Work out the finished part from the listing and answer in its coordinate system (mm). Face numbers are marked on the shaded views. A direction names the side the tool comes from. Give positions to 0.01 mm unless a question says otherwise; leave off trailing zeros. Write item = value, one per line. Start each with the question number.
1. Flat-ended cylindrical pins translate along their axes: pin 1 Ø4 at (x, z) = (34.5, -5) entering from +Y; pin 2 Ø8 at (x, y) = (35.5, -1.5) entering from +Z; pin 3 Ø4 at (x, y) = (33.5, 3) entering from +Z; pin 4 Ø8 at (y, z) = (-5.5, 0.5) entering from +X. Find the tip coordinate at first contact, or state that the pin passes through.
2. For the marked faces 1 and 2, determine the directions among +Z, -Z, +X, -X, +Y, -Y from which every point of the face is accessible in a straight line to the end or side of a thin tool.
3. Consider L1, parallel to X at y = 4, z = -2; L2, parallel to Z at x = 51, y = -3; L3, parallel to Y at x = 27, z = -5.25. Determine where each line is inside the solid, lowest interval first. Write a range as [from, to].
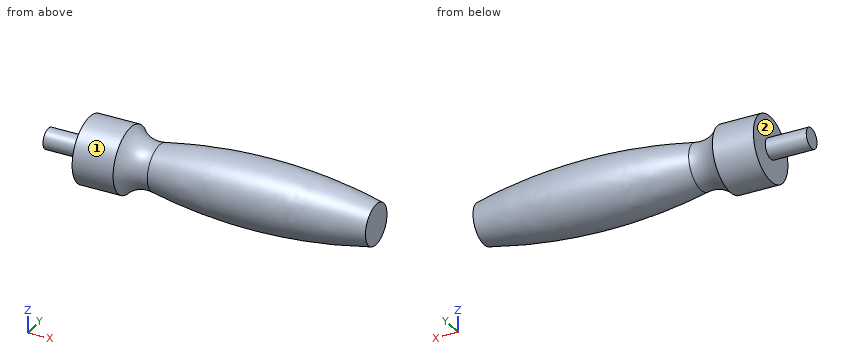
```python
from build123d import *

# Parameters (mm, degrees)
F0_W = 10
F0_H = 2.5


# Not quite as in the source:
# - a fillet or chamfer that OpenCascade refuses, or shapes differently, is made with other operations: its cross-section is extruded or revolved along the edge and cut away or added


with BuildPart() as f1:
    # F0 (on Front) → F1 (revolve)
    with BuildSketch(Plane.XZ):
        with Locations((-5, 1.25)):
            Rectangle(F0_W, F0_H)
        Polygon((0, 8), (0, 2.5), (0, 0), (10, 0), (10, 4), (10, 8), align=None)
        with BuildLine():
            Line((10, 4), (10, 0))
            Line((10, 0), (70, 0))
            Line((70, 0), (70, 5))
            ThreePointArc((70, 5), (39.9419698495, 7.9818090321), (10, 4))
        make_face()
    revolve(axis=Axis((40, 0, 0), (1, 0, 0)))

    # F2: fillet of radius 7.5 on 1 edges, made by hand

    # F2_s1 → F2_t2 (revolve)
    with BuildSketch(Plane.XZ):
        with BuildLine():
            ThreePointArc((17.0739020896, 5.582469697), (13.2142793321, 5.8470695986), (10, 8))
            Line((10, 8), (10, 4))
            ThreePointArc((10, 4), (13.5260036045, 4.8401717227), (17.0739020896, 5.582469697))
        make_face()
    revolve(axis=Axis((10, 0, 0), (1, 0, 0)))


solid = f1.part
```
Verdict:
q1.pin_1 = 7.19
q1.pin_2 = 7.97
q1.pin_3 = 7.68
q1.pin_4 = 70
q2.face_1 = +X, -X
q2.face_2 = -X
q3.L1 = [0, 70]
q3.L2 = [-7.09, 7.09]
q3.L3 = [-4.82, 4.82]
